Here's how the part is built. I have some questions about the finished solid (model axes, mm). A direction names the side the tool comes from. Round coordinates to 2 decimals unless told otherwise and drop trailing zeros. Loops run counter-clockwise (first coordinate to the right, second up) from the corner with the lowest first, then second, coordinate; pieces in that order, holes last. Notation, with made-up numbers: (67, 19.25) - (103, 19.25) arc R21 ccw to (103, 31.25) - close; hole circle Ø6 at (2.5, 8.5). An arc over 180 degrees is marked (long way). Answer as a JSON object with one key per item and string values. Group by question number.
1) If I drill on line 1 along Y through (x, z) = (13.25, 3.5); line 2 along X through (y, z) = (-1.5, 3.25); line 3 along X through (y, z) = (-4.75, 3.5), over which ranges is the centre line in solid material (lowest first)? Write a range as [from, to].
2) If we mould it in two halves opening along Y, with no side actions, what happens to faces 1 (the face through (17.145, 3.746, 4.93)), 2 (the face through (13, 3.1, 5)), 3 (the face through (15.8, -5.3, 4.9))? For each: pulls with the +Y half, pulls with the -Y half, needs draft (parallel to the pull), parting line crosses it, or undercut.
3) I want a section at C-C, the plane y = -2. Please give me the cut outline in (x, z), then the cut area to 3 significant figures.
4) Will these pins go through, and if not, where does the flat tip stop? P1, Ø1.6, axis at y = 5, z = 5.5, coming from the -X side; P2, Ø4, axis at x = 14.5, y = -1.5, coming from the -Z side; P3, Ø4, axis at x = 12, z = 6, coming from the -Y side; P4, Ø3, axis at y = -1, z = 3, coming from the -X side.
5) I want a section at B-B, the plane z = 2.5. Please give me the cut outline in (x, y), then the cut area to 3 significant figures.
6) I want a section at A-A, the plane x = 14.25. Please give me the cut outline in (y, z), then the cut area to 3 significant figures.
7) I want a section at D-D, the plane x = 15.75. Please give me the cut outline in (y, z), then the cut area to 3 significant figures.
8) Which directions (+Z, -Z, +X, -X, +Y, -Y) give clear straight access to the entire face, cutting with the end or side of a thin tool? Please do faces 4 (the face through (13, -3.1, 5)), 5 (the face through (17.15, -3.73, 4.93)), 6 (the face through (15, -5, 5)), 7 (the face through (14, 4.1, 5)).
Autodesk Inventor part; units mm, degrees
ref_plane "YZ Plane" through (0, 0, 0) normal (1, 0, 0) x (0, 1, 0)
ref_plane "XZ Plane" through (0, 0, 0) normal (0, 1, 0) x (-1, 0, 0)
ref_plane "XY Plane" through (0, 0, 0) normal (0, 0, 1) x (1, 0, 0)
sketch "Sketch1" plane through (0, 0, 0) normal (0, 0, 1) x (1, 0, 0)
  line L0 (15, -4.1) -> (12.1, -4.1)
  line L1 (12.1, 4.1) -> (15, 4.1)
  line L2 (12.1, 4.1) -> (12.1, 5.1)
  line L3 (10.3015, 3.1) -> (12.1, 5.1)
  line L4 (10.3015, -3.1) -> (12.1, -5.1)
  line L5 (12.1, -5.1) -> (12.1, -4.1)
  line L6 (15.3015, 3.1) -> (15.3015, -3.1)
  line L7 (15, 4.1) -> (15, 6.1)
  line L8 (15, 6.1) -> (16.7157, 4.3843)
  line L9 (15, -4.1) -> (15, -6.1)
  line L10 (15, -6.1) -> (16.7157, -4.3843)
  line L11 (17.3015, 2.97) -> (17.3015, -2.97)
  line L12 (15.3015, 3.1) -> (10.3015, 3.1)
  line L13 (15.3015, -3.1) -> (10.3015, -3.1)
  arc A0 (17.3015, 2.97) -> (16.7157, 4.3843) centre (15.3015, 2.97) ccw
  arc A1 (16.7157, -4.3843) -> (17.3015, -2.97) centre (15.3015, -2.97) ccw
  point P0 (0, 0)
  point P1 (17.3015, 3.7985)
  point P2 (17.3015, -3.7985)
  dimension "d0" = 1
  dimension "d2" = 45
  dimension "d3" = 45
  dimension "d4" = 2.3015
  dimension "d5" = 2.3015
  dimension "d6" = 2
  dimension "d7" = 2
  dimension "d8" = 1
  dimension "d9" = 1
  dimension "d10" = 5
  dimension "d11" = 5
  dimension "d12" = 1
  dimension "d13" = 2
  dimension "d16" = 2.9
  dimension "d17" = 2.9
  dimension "d18" = 2
extrude "Extrusion1" add sketch "Sketch1" along normal blind 10
equation "\"d7\" = d6"
equation "\"d9\" = d8"
equation "\"d11\" = d10"
equation "\"d12\" = d0"
equation "\"d17\" = d16"
properties part number "clema cablu profil"
Outcome:
{
 "1": {"line 1": "[-4.1, -3.1], [3.1, 4.1]", "line 2": "[15.3, 17.3]", "line 3": "[11.79, 12.1], [15, 16.35]"},
 "2": {"face 1": "pulls with the +Y half", "face 2": "undercut", "face 3": "pulls with the -Y half"},
 "3": {"outline": "(15.3, 0) - (17.3, 0) - (17.3, 10) - (15.3, 10) - close", "area": "20.0 mm^2"},
 "4": {"P1": "x = 11.29", "P2": "z = 0", "P3": "y = -5.1", "P4": "x = 15.3"},
 "5": {"outline": "(10.3, -3.1) - (12.1, -5.1) - (12.1, -4.1) - (15, -4.1) - (15, -6.1) - (16.72, -4.38) arc R2 ccw to (17.3, -2.97) - (17.3, 2.97) arc R2 ccw to (16.72, 4.38) - (15, 6.1) - (15, 4.1) - (12.1, 4.1) - (12.1, 5.1) - (10.3, 3.1) - (15.3, 3.1) - (15.3, -3.1) - close", "area": "30.1 mm^2"},
 "6": {"outline": "(-4.1, 0) - (-3.1, 0) - (-3.1, 10) - (-4.1, 10) - close; (3.1, 0) - (4.1, 0) - (4.1, 10) - (3.1, 10) - close", "area": "20.0 mm^2"},
 "7": {"outline": "(-5.35, 0) - (5.35, 0) - (5.35, 10) - (-5.35, 10) - close", "area": "107 mm^2"},
 "8": {"face 4": "+Z, -Z, -X", "face 5": "+Z, -Z, +X, -Y", "face 6": "+Z, -Z, -Y", "face 7": "+Z, -Z, +Y"}
}
